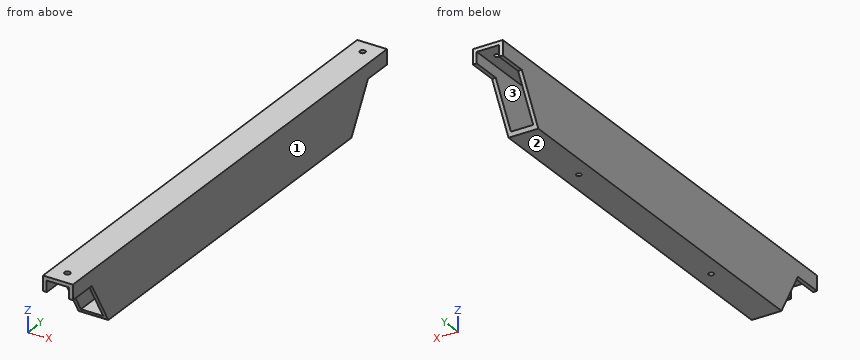
from build123d import *

# Parameters (mm, degrees)
SKETCH1_W              = 25.4
SKETCH1_H              = 50.8
SKETCH1_W_2            = 19.05
SKETCH1_H_2            = 44.45
BOSS_EXTRUDE1_DEPTH    = 419.1
F_10_CLEARANCE_HOLE1_D = 4.7625
CUT_EXTRUDE1_DEPTH     = 423.930975456
CUT_EXTRUDE2_REACH     = 424.931
SKETCH6_R              = 2.1828125


with BuildPart() as part:
    # Sketch1 → Boss-Extrude1 (new body)
    with BuildSketch(Plane(origin=(0, 0, 0), x_dir=(1, 0, 0), z_dir=(0, 1, 0))):
        with Locations((12.7, 25.4)):
            Rectangle(SKETCH1_W, SKETCH1_H)
        with Locations((12.7, 25.4)):
            Rectangle(SKETCH1_W_2, SKETCH1_H_2, mode=Mode.SUBTRACT)
    extrude(amount=BOSS_EXTRUDE1_DEPTH)

    # #10 Clearance Hole1 (through all)
    with Locations(Plane(origin=(0, 0, -50.8), x_dir=(-1, 0, 0), z_dir=(0, 0, -1))):
        with Locations((-12.7, 406.4), (-12.7, 12.7)):
            Hole(F_10_CLEARANCE_HOLE1_D / 2)

    # Sketch5 → Cut-Extrude1 (cut, through all)
    with BuildSketch(Plane(origin=(25.4, 0, 0), x_dir=(0, 0, -1), z_dir=(1, 0, 0))):
        Polygon((12.7, 419.1), (12.7, 393.7), (50.8, 371.702954744), (50.8, 419.1), align=None)
    cut_extrude1 = extrude(amount=-CUT_EXTRUDE1_DEPTH, mode=Mode.SUBTRACT)

    # Mirror1: Cut-Extrude1 across plane
    add(cut_extrude1.mirror(Plane.ZX.offset(209.55)), mode=Mode.SUBTRACT)

    # Sketch6 → Cut-Extrude2 (cut, up to next)
    with BuildSketch(Plane(origin=(0, 0, -50.8), x_dir=(-1, 0, 0), z_dir=(0, 0, -1)), mode=Mode.PRIVATE) as cut_extrude2_sk1:
        with Locations((-12.7, 121.2725)):
            Circle(SKETCH6_R)
    cut_extrude2_tool1 = extrude(cut_extrude2_sk1.sketch, amount=-CUT_EXTRUDE2_REACH, mode=Mode.PRIVATE) & part.part
    # Sketch6 → Cut-Extrude2 (cut, up to next)
    with BuildSketch(Plane(origin=(0, 0, -50.8), x_dir=(-1, 0, 0), z_dir=(0, 0, -1)), mode=Mode.PRIVATE) as cut_extrude2_sk2:
        with Locations((-12.7, 297.8275)):
            Circle(SKETCH6_R)
    cut_extrude2_tool2 = extrude(cut_extrude2_sk2.sketch, amount=-CUT_EXTRUDE2_REACH, mode=Mode.PRIVATE) & part.part
    add(cut_extrude2_tool1.solids().sort_by_distance((12.7, 121.2725, -50.8))[0], mode=Mode.SUBTRACT)
    add(cut_extrude2_tool2.solids().sort_by_distance((12.7, 297.8275, -50.8))[0], mode=Mode.SUBTRACT)


solid = part.part
Model file for the job. Use its own axes, mm. Face numbers are marked on the shaded views. Give positions to 0.01 mm unless a question says otherwise; leave off trailing zeros. Loops run counter-clockwise (first coordinate to the right, second up) from the corner with the lowest first, then second, coordinate; pieces in that order, holes last.
1) Saw through at A-A (x = 18.5). Write the cut outline in (y, z) (3 decimals), plus the area to 3 significant figures.
2) Saw through at C-C (z = -25). Write the cut outline in (x, y) (3 decimals).
3) Pull direction X, two halves, no side cores. Call the marked faces 1, 2 and 3: +X half, -X half, draft (parallel to the pull), parting line (faces both ways), or undercut.
4) Wall check: line 1 (Y direction, x = 12.7, z = -2.45); line 2 (X direction, y = 134.5, z = -12) (3 decimals); line 3 (Z direction, x = 4, y = 313) (3 decimals). Give the ranges that are in metal, low to high.
5) Saw through at B-B (y = 275). Write the cut outline in (x, z) (3 decimals).
6) Flat gauge pins, fed straight in: pin 1 Ø1.6 at (x, y) = (1, 6.5) entering from -Z; pin 2 Ø6 at (x, y) = (12.7, 12.7) entering from -Z (3 decimals). Where does each tip first touch, or does it go through?
Answer block:
1. outline: (0, -3.175) - (419.1, -3.175) - (419.1, 0) - (0, 0) - close; (45.564, -47.625) - (47.397, -50.8) - (371.703, -50.8) - (373.536, -47.625) - close
1. area: 2,370 mm2
2. outline: (0, 32.501) - (3.175, 32.501) - (3.175, 386.599) - (0, 386.599) - close; (22.225, 32.501) - (25.4, 32.501) - (25.4, 386.599) - (22.225, 386.599) - close
3. face 1: +X half
3. face 2: draft
3. face 3: undercut
4. line 1: y = 0 to 10.32, 15.08 to 404.02, 408.78 to 419.1
4. line 2: x = 0 to 3.175, 22.225 to 25.4
4. line 3: z = -50.8 to -47.625, -3.175 to 0
5. outline: (0, -50.8) - (25.4, -50.8) - (25.4, 0) - (0, 0) - close; hole (3.175, -47.625) - (22.225, -47.625) - (22.225, -3.175) - (3.175, -3.175) - close
6. pin 1: stops at z = -12.7
6. pin 2: stops at z = -3.175
